Input: part model. Units: mm. Frame: model coordinates. A direction names the side the tool comes from. Coordinates: 2 decimals unless noted, no trailing zeros. Write each loop counter-clockwise with the first axis right and the second up, starting at its lowest first coordinate (ties: lowest second). Pieces come first, ordered by that corner, then holes. Notation, with made-up numbers: M -30.5,51.25 L 16.5,51.25 A25 ccw 16.5,63.25 Z; hole C 54.5,16 d4. An arc over 180 degrees is marked long. Use one line per item in the form item = value.
from build123d import *

# Parameters (mm, degrees)
SKETCH_1_R           = 19
EXTRUDE_1_DEPTH      = 80
SKETCH_2_W           = 8
SKETCH_2_H           = 8
EXTRUDE_2_DEPTH      = 0.1
EXTRUDE_2_DEPTH_BACK = 60
SKETCH_3_R           = 175
EXTRUDE_3_DEPTH      = 19
SKETCH_4_R           = 125
SKETCH_4_R_2         = 118
EXTRUDE_4_DEPTH      = 5
SKETCH_5_R           = 118
SKETCH_5_R_2         = 40
CUT_EXTRUDE_1_DEPTH  = 10
CHAMFER_1_SIZE       = 1
SKETCH_6_R           = 9.5
CUT_EXTRUDE_2_DEPTH  = 20
SKETCH_7_R           = 110
EXTRUDE_5_DEPTH      = 55
SKETCH_8_R           = 116
EXTRUDE_6_DEPTH      = 204
SKETCH_9_R           = 120
EXTRUDE_7_DEPTH      = 102
CHAMFER_2_SIZE       = 45
EXTRUDE_8_DEPTH      = 170
CUT_EXTRUDE_3_REACH  = 309
SKETCH_11_R          = 9.5
SKETCH_12_W          = 86
SKETCH_12_H          = 86
EXTRUDE_9_DEPTH      = 193
SKETCH_13_R          = 32
EXTRUDE_10_DEPTH     = 126
CHAMFER_3_SIZE       = 1
SKETCH_15_R          = 7
SKETCH_16_R          = 15
EXTRUDE_11_DEPTH     = 10
EXTRUDE_12_DEPTH     = 15
SKETCH_18_R          = 8
CUT_EXTRUDE_4_DEPTH  = 15


with BuildPart() as part:
    # Эскиз1 → Вытянуть1 (new body)
    with BuildSketch(Plane.XY):
        Circle(SKETCH_1_R)
    extrude(amount=EXTRUDE_1_DEPTH)

    # Эскиз2 → Вытянуть2 (add, two sides)
    with BuildSketch(Plane(origin=(0, 0, 0), x_dir=(-1, 0, 0), z_dir=(0, 0, -1))) as extrude_2_sk:
        with Locations((0, 18)):
            Rectangle(SKETCH_2_W, SKETCH_2_H)
    extrude(amount=EXTRUDE_2_DEPTH)
    extrude(extrude_2_sk.sketch, amount=-EXTRUDE_2_DEPTH_BACK)

    # Эскиз3 → Вытянуть3 (add)
    with BuildSketch(Plane.XY.offset(80)):
        Circle(SKETCH_3_R)
    extrude(amount=EXTRUDE_3_DEPTH)

    # Эскиз4 → Вытянуть4 (add)
    with BuildSketch(Plane(origin=(0, 0, 80), x_dir=(-1, 0, 0), z_dir=(0, 0, -1))):
        with Locations(Location((0, 0, 0), (0, 0, 180))):  # turned: the seam where the file's is
            Circle(SKETCH_4_R)
        Circle(SKETCH_4_R_2, mode=Mode.SUBTRACT)
    extrude(amount=EXTRUDE_4_DEPTH)

    # Эскиз5 → Вырез-Вытянуть1 (cut)
    with BuildSketch(Plane(origin=(0, 0, 80), x_dir=(-1, 0, 0), z_dir=(0, 0, -1))):
        Circle(SKETCH_5_R)
        Circle(SKETCH_5_R_2, mode=Mode.SUBTRACT)
    extrude(amount=-CUT_EXTRUDE_1_DEPTH, mode=Mode.SUBTRACT)

    # Фаска1
    chamfer_1_edges = [part.edges().sort_by_distance(p)[0] for p in [
        (-125, 0, 75),
        (40, 0, 80),
        (-11.937336386, -14.781745499, 0),
    ]]
    chamfer(chamfer_1_edges, length=CHAMFER_1_SIZE)

    # Эскиз6 → Вырез-Вытянуть2 (cut, through all)
    with BuildSketch(Plane(origin=(0, 0, 80), x_dir=(-1, 0, 0), z_dir=(0, 0, -1))):
        with Locations((-57.402514855, 138.581929877)):
            Circle(SKETCH_6_R)
        with Locations((57.402514855, 138.581929877)):
            Circle(SKETCH_6_R)
        with Locations((138.581929877, 57.402514855)):
            Circle(SKETCH_6_R)
        with Locations((138.581929877, -57.402514855)):
            Circle(SKETCH_6_R)
        with Locations((57.402514855, -138.581929877)):
            Circle(SKETCH_6_R)
        with Locations((-57.402514855, -138.581929877)):
            Circle(SKETCH_6_R)
        with Locations((-138.581929877, -57.402514855)):
            Circle(SKETCH_6_R)
        with Locations((-138.581929877, 57.402514855)):
            Circle(SKETCH_6_R)
    extrude(amount=-CUT_EXTRUDE_2_DEPTH, mode=Mode.SUBTRACT)

    # Эскиз7 → Вытянуть5 (add)
    with BuildSketch(Plane.XY.offset(99)):
        Circle(SKETCH_7_R)
    extrude(amount=EXTRUDE_5_DEPTH)

    # Эскиз8 → Вытянуть6 (add)
    with BuildSketch(Plane.XY.offset(154)):
        Circle(SKETCH_8_R)
    extrude(amount=EXTRUDE_6_DEPTH)

    # Эскиз9 → Вытянуть7 (add)
    with BuildSketch(Plane.XY.offset(358)):
        Circle(SKETCH_9_R)
    extrude(amount=EXTRUDE_7_DEPTH)

    # Фаска2
    chamfer_2_edges = [part.edges().sort_by_distance(p)[0] for p in [
        (-120, 0, 460),
    ]]
    chamfer(chamfer_2_edges, length=CHAMFER_2_SIZE)

    # Эскиз10 → Вытянуть8 (add)
    with BuildSketch(Plane(origin=(0, 0, 154), x_dir=(-1, 0, 0), z_dir=(0, 0, -1))):
        Polygon((-123, -132), (-83.762395693, -132), (-58.16412012, -87.662486121), (-72.020526581, -79.662486121), (-93, -116), (-123, -116), align=None)
        Polygon((123, -132), (83.762395693, -132), (58.16412012, -87.662486121), (72.020526581, -79.662486121), (93, -116), (123, -116), align=None)
    extrude(amount=-EXTRUDE_8_DEPTH)

    # Эскиз11 → Вырез-Вытянуть3 (cut, up to next)
    with BuildSketch(Plane.XZ.offset(132), mode=Mode.PRIVATE) as cut_extrude_3_sk1:
        with Locations((-108, 169)):
            Circle(SKETCH_11_R)
    cut_extrude_3_tool1 = extrude(cut_extrude_3_sk1.sketch, amount=-CUT_EXTRUDE_3_REACH, mode=Mode.PRIVATE) & part.part
    add(cut_extrude_3_tool1.solids().sort_by_distance((-108, -132, 169))[0], mode=Mode.SUBTRACT)
    # Эскиз11 → Вырез-Вытянуть3 (cut, up to next)
    with BuildSketch(Plane.XZ.offset(132), mode=Mode.PRIVATE) as cut_extrude_3_sk2:
        with Locations((108, 169)):
            Circle(SKETCH_11_R)
    cut_extrude_3_tool2 = extrude(cut_extrude_3_sk2.sketch, amount=-CUT_EXTRUDE_3_REACH, mode=Mode.PRIVATE) & part.part
    add(cut_extrude_3_tool2.solids().sort_by_distance((108, -132, 169))[0], mode=Mode.SUBTRACT)
    # Эскиз11 → Вырез-Вытянуть3 (cut, up to next)
    with BuildSketch(Plane.XZ.offset(132), mode=Mode.PRIVATE) as cut_extrude_3_sk3:
        with Locations((-108, 309)):
            Circle(SKETCH_11_R)
    cut_extrude_3_tool3 = extrude(cut_extrude_3_sk3.sketch, amount=-CUT_EXTRUDE_3_REACH, mode=Mode.PRIVATE) & part.part
    add(cut_extrude_3_tool3.solids().sort_by_distance((-108, -132, 309))[0], mode=Mode.SUBTRACT)
    # Эскиз11 → Вырез-Вытянуть3 (cut, up to next)
    with BuildSketch(Plane.XZ.offset(132), mode=Mode.PRIVATE) as cut_extrude_3_sk4:
        with Locations((108, 309)):
            Circle(SKETCH_11_R)
    cut_extrude_3_tool4 = extrude(cut_extrude_3_sk4.sketch, amount=-CUT_EXTRUDE_3_REACH, mode=Mode.PRIVATE) & part.part
    add(cut_extrude_3_tool4.solids().sort_by_distance((108, -132, 309))[0], mode=Mode.SUBTRACT)

    # Эскиз12 → Вытянуть9 (add)
    with BuildSketch(Plane(origin=(0, 0, 0), x_dir=(1, 0, 0), z_dir=(0, 1, 0))):
        with Locations((0, -198)):
            Rectangle(SKETCH_12_W, SKETCH_12_H)
    extrude(amount=EXTRUDE_9_DEPTH)

    # Эскиз13 → Вытянуть10 (add)
    with BuildSketch(Plane(origin=(0, 0, 0), x_dir=(1, 0, 0), z_dir=(0, 1, 0))):
        with Locations(Location((0, -286, 0), (0, 0, 90))):  # turned: the seam where the file's is
            Circle(SKETCH_13_R)
    extrude(amount=EXTRUDE_10_DEPTH)

    # Фаска3
    chamfer_3_edges = [part.edges().sort_by_distance(p)[0] for p in [
        (0, 126, 318),
    ]]
    chamfer(chamfer_3_edges, length=CHAMFER_3_SIZE)

    # По траектории1: sweep along a path in Эскиз14
    with BuildLine(Plane.XY.offset(286)) as sweep_1_path:
        CenterArc((0, 152), 26, 0, 360)
    # Эскиз15 → По траектории1 (sweep)
    with BuildSketch(Plane(origin=(0, 0, 0), x_dir=(0, 0, -1), z_dir=(1, 0, 0))):
        with Locations((-286, 178)):
            Circle(SKETCH_15_R)
    sweep(path=sweep_1_path.line)

    # Эскиз16 → Вытянуть11 (add)
    with BuildSketch(Plane.ZY.offset(43)):
        with Locations(Location((198, 150, 0), (0, 0, 180))):  # turned: the seam where the file's is
            Circle(SKETCH_16_R)
    extrude(amount=EXTRUDE_11_DEPTH)

    # Эскиз17 → Вытянуть12 (add)
    with BuildSketch(Plane.ZY.offset(53)):
        Polygon((198, 172.516660498), (178.5, 161.258330249), (178.5, 138.741669751), (198, 127.483339502), (217.5, 138.741669751), (217.5, 161.258330249), align=None)
    extrude(amount=EXTRUDE_12_DEPTH)

    # Эскиз18 → Вырез-Вытянуть4 (cut)
    with BuildSketch(Plane.ZY.offset(68)):
        with Locations((198, 150)):
            Circle(SKETCH_18_R)
    extrude(amount=-CUT_EXTRUDE_4_DEPTH, mode=Mode.SUBTRACT)


solid = part.part
(1) Line query: probe 1 along Z at (x, y) = (-108, -125.75); probe 2 along Y at (x, z) = (-130.5, 80.5); probe 3 along Z at (x, y) = (133, 7). Output: solid intervals per line, ascending.
Computed:
probe_1 = 80 to 99, 154 to 159.5, 178.5 to 299.5, 318.5 to 324
probe_2 = -116.6 to -62.4, -52.41 to 52.41, 62.4 to 116.6
probe_3 = 80 to 99
(2) Pull-direction query (X, two-part tool) for faces 1 (the cylindrical face through (-128.982, 118.273, 89.367)), 2 (the flat face through (104, -132, 238)), 3 (the cylindrical face through (59.462, 129.308, 89.367)), 4 (the cylindrical face through (105.941, -124.112, 299.726)); classes: pulls with the +X half, pulls with the -X half, needs draft (parallel to the pull), parting line crosses it, or undercut.
Computed:
face_1 = parting line crosses it
face_2 = needs draft
face_3 = undercut
face_4 = undercut
(3) Set-up query: faces 5 (the flat face through (-2, -114, 99)), 6 (the flat face through (-60, 150, 178.5)), 7 (the flat face through (-119, 41, 80)). Return all of +Z, -Z, +X, -X, +Y, -Y with unobstructed straight access to the full face (end or side cutting, diameter ignored); none if empty.
Computed:
face_5 = none
face_6 = -X, +Y
face_7 = -Z
(4) Section query A-A on z = 169. Return the cut outline in (x, y), plus the area to 3 significant figures.
Computed:
outline = M -123,-132 L -117.5,-132 L -117.5,-116 L -123,-116 Z; M -98.5,-132 L -83.76,-132 L -63.57,-97.03 A116 ccw 63.57,-97.03 L 83.76,-132 L 98.5,-132 L 98.5,-116 L 93,-116 L 76.42,-87.27 A116 ccw 43,107.74 L 43,193 L -43,193 L -43,107.74 A116 ccw -76.42,-87.27 L -93,-116 L -98.5,-116 Z; M 117.5,-132 L 123,-132 L 123,-116 L 117.5,-116 Z
area = 50,800 mm^2
(5) First-contact query: pin 1 Ø22 at (x, y) = (57.4, -138.58) entering from -Z; pin 2 Ø6.5 at (y, z) = (17, 17) entering from +X; pin 3 Ø17.5 at (y, z) = (147.5, 199) entering from -X. Flat tips, straight axial feed; report the tip coordinate or a pass-through.
Computed:
pin_1 = 80
pin_2 = 13.11
pin_3 = -68
(6) Section query C-C on z = 405.5. Return the cut outline in (x, y).
Computed:
outline = C 0,0 d240
(7) Section query B-B on x = 135. Return the cut outline in (y, z), plus the area to 3 significant figures.
Computed:
outline = M -111.36,80 L -66.2,80 L -66.2,99 L -111.36,99 Z; M -48.6,80 L 48.6,80 L 48.6,99 L -48.6,99 Z; M 66.2,80 L 111.36,80 L 111.36,99 L 66.2,99 Z
area = 3,560 mm^2
